Read the model definition and answer for the solid it produces. Units are mm, in the model's axes. Face numbers are marked on the shaded views. Coordinates: 2 decimals unless noted, no trailing zeros. Write each loop counter-clockwise with the first axis right and the second up, starting at its lowest first coordinate (ties: lowest second). Pieces come first, ordered by that corner, then holes.
Item 1: Section A-A (x = -3.5) is taken. Give the vertices of the cut face in (y, z), then the cut area to 3 significant figures.
Item 2: Section D-D (x = 0) is taken. Give the vertices of the cut face in (y, z).
Item 3: Each of these flat-tipped pins is pushed along its axis until it touches: P1, Ø1.5, axis at x = -6.5, y = 8, coming from the +Z side; P2, Ø6, axis at y = 12, z = -9.5, coming from the -X side; P3, Ø1.5, axis at y = 15.5, z = -8.5, coming from the -X side; P4, Ø10, axis at y = 7, z = 4, coming from the +X side. Where does it stop, or does it pass through?
Item 4: Straight lines are drawn through the part: probe 1 along X at (y, z) = (37, 0); probe 2 along Z at (x, y) = (2, 4); probe 3 along Z at (x, y) = (6, 26). For each, find the intervals that lie inside material, in ascending order.
Item 5: Section B-B (z = 10) is taken. Give the vertices of the cut face in (x, y).
Item 6: Section C-C (y = 23) is taken. Give the vertices of the cut face in (x, z), then the cut area to 3 significant figures.
Item 7: Determine the mould class of the marked faces 1, 2 and 3 for opening direction X: released by +X, released by -X, zero draft, split by the parting line, or undercut.
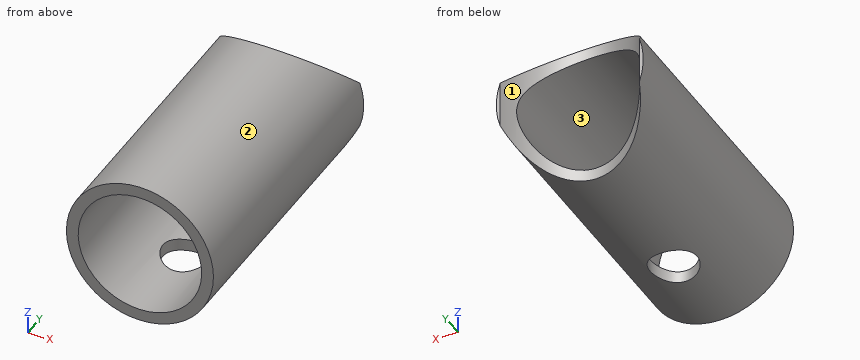
from build123d import *

# Parameters (mm, degrees)
SKETCH_1_R               = 12.5
SKETCH_1_R_2             = 10.5
EXTRUDE_1_DEPTH          = 48.5
CUT_EXTRUDE_1_DEPTH      = 52.621216568
CUT_EXTRUDE_1_DEPTH_BACK = 52.621216568
SKETCH_2_R               = 12.5
SKETCH_3_R               = 4
CUT_EXTRUDE_2_DEPTH      = 52.621216687


with BuildPart() as part:
    # Эскиз1 → Бобышка-Вытянуть1 (new body)
    with BuildSketch(Plane(origin=(0, 0, 0), x_dir=(1, 0, 0), z_dir=(0, 1, 0))):
        with Locations(Location((0, 0, 0), (0, 0, 90))):
            Circle(SKETCH_1_R)
        with Locations(Location((0, 0, 0), (0, 0, 90))):
            Circle(SKETCH_1_R_2, mode=Mode.SUBTRACT)
    extrude(amount=EXTRUDE_1_DEPTH)

    # Эскиз2 → Вырез-Вытянуть1 (cut, two sides: drawn at the far end of the back side and taken through both)
    with BuildSketch(Plane.XY.offset(-CUT_EXTRUDE_1_DEPTH_BACK)):
        with Locations((0, 52.5)):
            Circle(SKETCH_2_R)
    extrude(amount=CUT_EXTRUDE_1_DEPTH + CUT_EXTRUDE_1_DEPTH_BACK, mode=Mode.SUBTRACT)

    # Эскиз3 → Вырез-Вытянуть2 (cut, through all)
    with BuildSketch(Plane.XY):
        with Locations(Location((0, 15, 0), (0, 0, 90))):
            Circle(SKETCH_3_R)
    extrude(amount=-CUT_EXTRUDE_2_DEPTH, mode=Mode.SUBTRACT)


solid = part.part
Established:
1. outline: (0, -12) - (13.06, -12) - (13.06, -9.9) - (0, -9.9) - close; (0, 9.9) - (40.5, 9.9) - (40.5, 12) - (0, 12) - close; (16.94, -12) - (40.5, -12) - (40.5, -9.9) - (16.94, -9.9) - close
1. area: 162 mm2
2. outline: (0, -12.5) - (11, -12.5) - (11, -10.5) - (0, -10.5) - close; (0, 10.5) - (40, 10.5) - (40, 12.5) - (0, 12.5) - close; (19, -12.5) - (40, -12.5) - (40, -10.5) - (19, -10.5) - close
3. P1: stops at z = 11.1
3. P2: stops at x = -10.68
3. P3: stops at x = -9.81
3. P4: stops at x = 12.5
4. probe 1: x = -12.5 to -10.5, 10.5 to 12.5
4. probe 2: z = -12.34 to -10.31, 10.31 to 12.34
4. probe 3: z = -10.97 to -8.62, 8.62 to 10.97
5. outline: (-7.5, 0) - (-3.2, 0) - (-3.2, 40.42) arc R12.5 cw to (-7.5, 42.5) - close; (3.2, 0) - (7.5, 0) - (7.5, 42.5) arc R12.5 cw to (3.2, 40.42) - close
6. outline: circle Ø25 at (0, 0); hole circle Ø21 at (0, 0)
6. area: 145 mm2
7. face 1: undercut
7. face 2: split by the parting line
7. face 3: undercut
